Design review of the part built by this model. Coordinates are the model's own, in mm. Face numbers are marked on the shaded views. A direction names the side the tool comes from. Give positions to 0.01 mm unless a question says otherwise; leave off trailing zeros. Loops run counter-clockwise (first coordinate to the right, second up) from the corner with the lowest first, then second, coordinate; pieces in that order, holes last. Notation, with made-up numbers: (0.25, 56.25) -> (47.25, 56.25) arc R10 cw to (47.25, 72.25) -> close; hole circle Ø8 at (15, 72.5). An arc over 180 degrees is marked (long way). Use CSV: the item, a comma, the result in double quotes. Start each with the question number.
Item 1: Wall thickness on line 1 along X through (y, z) = (5, 18.5) (3 decimals); line 2 along Y through (x, z) = (-30, 10.75); line 3 along X through (y, z) = (-1, 2): over which ranges is each line inside the solid? List them lowest first. Write a range as from..to.
Item 2: The part is to be moulded in two halves that separate along X. For the marked faces 1, 2, 3 and 4, say which applies: +X half, -X half, draft (parallel to the pull), parting line (faces both ways), or undercut.
Item 3: We need section C-C (z = 26). State the section outline as (x, y) points.
Item 4: We need section D-D (z = 6.5). Count the separate pieces of the cut face and the enclosed holes in it, plus the area to 3 significant figures.
Item 5: Clearance check with flat-ended pins moving along their axes: pin 1 (8 mm diameter, centred on x = -31.5, y = -1, fed in from -Z); pin 2 (7 mm diameter, centred on x = 30, y = 0, fed in from -Z); pin 3 (7 mm diameter, centred on x = 0.5, y = -2, fed in from +Z); pin 4 (1.7 mm diameter, centred on x = 38.02, y = -8.92, fed in from -Z). State where each tip first meets the part, or that it passes through.
Item 6: For the marked faces 5 and 6, list the 3-axis set-ups (+Z, -Z, +X, -X, +Y, -Y) from which the entire face can be reached by the end or side of a thin tool; tool diameter is ignored.
Item 7: We need section B-B (y = 0). State the section outline as (x, z) points.
Item 8: We need section A-A (x = 0). State the section outline as (y, z) points.
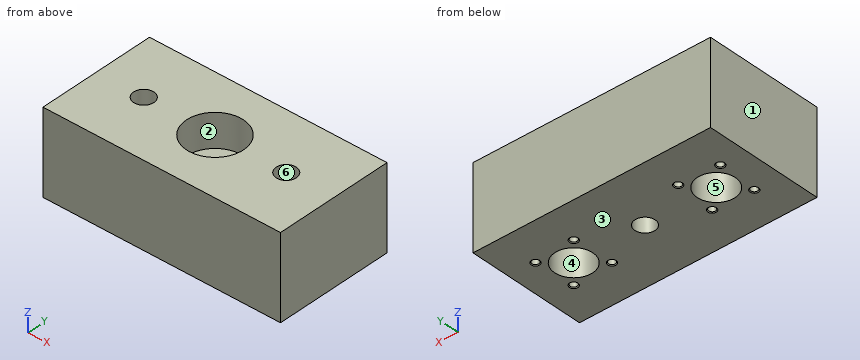
from build123d import *

# Parameters (mm, degrees)
SKETCH_1_W                     = 100
SKETCH_1_H                     = 50
EXTRUDE_1_DEPTH                = 35
HOLE_WIZARD_8_5_8_5_1_D        = 8.5
HOLE_WIZARD_1_D                = 24
HOLE_WIZARD_1_DEPTH            = 14
HOLE_WIZARD_2_D                = 8.5
HOLE_WIZARD_3_D                = 16
HOLE_WIZARD_3_DEPTH            = 20
HOLE_WIZARD_M3_5_1_D           = 2.9
HOLE_WIZARD_M3_5_1_DEPTH       = 10
HOLE_WIZARD_M3_5_1_CSINK_D     = 3.55
HOLE_WIZARD_M3_5_1_CSINK_ANGLE = 90
HOLE_WIZARD_M3_5_1_TIP         = 0.871247898


with BuildPart() as part:
    # 草图1 → 凸台-拉伸1 (new body)
    with BuildSketch(Plane.XY):
        Rectangle(SKETCH_1_W, SKETCH_1_H)
    extrude(amount=EXTRUDE_1_DEPTH)

    # Ø8.5 (8.5) 直径孔1 (through all)
    with Locations(Plane.XY.offset(35)):
        with Locations((0, 0)):
            Hole(HOLE_WIZARD_8_5_8_5_1_D / 2)

    # 孔1
    with Locations(Plane.XY.offset(35)):
        with Locations((0, 0)):
            Hole(HOLE_WIZARD_1_D / 2, depth=HOLE_WIZARD_1_DEPTH)

    # 孔2 (through all)
    with Locations(Plane(origin=(0, 0, 0), x_dir=(-1, 0, 0), z_dir=(0, 0, -1))):
        with Locations((30, 0)):
            hole_wizard_2 = Hole(HOLE_WIZARD_2_D / 2)

    # 镜向1: 孔2 across plane
    add(hole_wizard_2.mirror(Plane.ZY), mode=Mode.SUBTRACT)

    # 孔3
    with Locations(Plane(origin=(0, 0, 0), x_dir=(-1, 0, 0), z_dir=(0, 0, -1))):
        with Locations((30, 0), (-30, 0)):
            Hole(HOLE_WIZARD_3_D / 2, depth=HOLE_WIZARD_3_DEPTH)

    # M3.5 螺纹孔1
    with Locations(Plane(origin=(0, 0, 0), x_dir=(-1, 0, 0), z_dir=(0, 0, -1))):
        with Locations((21.077002862, -8.023722457), (38.023722457, -8.922997138), (38.922997138, 8.023722457), (21.976277543, 8.922997138), (-21.077002862, -8.023722457), (-38.023722457, -8.922997138), (-38.922997138, 8.023722457), (-21.976277543, 8.922997138)):
            CounterSinkHole(HOLE_WIZARD_M3_5_1_D / 2, HOLE_WIZARD_M3_5_1_CSINK_D / 2, depth=HOLE_WIZARD_M3_5_1_DEPTH, counter_sink_angle=HOLE_WIZARD_M3_5_1_CSINK_ANGLE)
            with Locations((0, 0, -(HOLE_WIZARD_M3_5_1_DEPTH + HOLE_WIZARD_M3_5_1_TIP / 2))):  # 118° drill point
                Cone(0, HOLE_WIZARD_M3_5_1_D / 2, HOLE_WIZARD_M3_5_1_TIP, mode=Mode.SUBTRACT)


solid = part.part
Results found:
1,line 1,"-50..-36.245, -23.755..23.755, 36.245..50"
1,line 2,"-25..-8, 8..25"
1,line 3,"-50..-37.94, -22.06..-4.13, 4.13..22.06, 37.94..50"
2,face 1,"-X half"
2,face 2,"undercut"
2,face 3,"draft"
2,face 4,"undercut"
3,outline,"(-50, -25) -> (50, -25) -> (50, 25) -> (-50, 25) -> close; hole circle Ø8.5 at (-30, 0); hole circle Ø24 at (0, 0); hole circle Ø8.5 at (30, 0)"
4,separate pieces,"1"
4,enclosed holes,"11"
4,area,"4,490 mm²"
5,pin 1,"z = 20"
5,pin 2,"through"
5,pin 3,"z = 21"
5,pin 4,"z = 10.36"
6,face 5,"-Z"
6,face 6,"+Z, -Z"
7,outline,"(-50, 0) -> (-38, 0) -> (-38, 20) -> (-34.25, 20) -> (-34.25, 35) -> (-50, 35) -> close; (-25.75, 20) -> (-22, 20) -> (-22, 0) -> (-4.25, 0) -> (-4.25, 21) -> (-12, 21) -> (-12, 35) -> (-25.75, 35) -> close; (4.25, 0) -> (22, 0) -> (22, 20) -> (25.75, 20) -> (25.75, 35) -> (12, 35) -> (12, 21) -> (4.25, 21) -> close; (34.25, 20) -> (38, 20) -> (38, 0) -> (50, 0) -> (50, 35) -> (34.25, 35) -> close"
8,outline,"(-25, 0) -> (-4.25, 0) -> (-4.25, 21) -> (-12, 21) -> (-12, 35) -> (-25, 35) -> close; (4.25, 0) -> (25, 0) -> (25, 35) -> (12, 35) -> (12, 21) -> (4.25, 21) -> close"
